Can you work these out from the drawing? Everything is in mm from the part's minimum corner. Give positions to 0.01 mm unless a question says otherwise; leave off trailing zeros. Loops run counter-clockwise (first coordinate to the right, second up) from the corner with the lowest first, then second, coordinate; pieces in that order, holes last. Notation, with made-up numbers: (-28.5, -0.75) -> (22.5, -0.75) arc R19 ccw to (22.5, 17.25) -> close; hole circle Ø7 at (6.25, -6.5). An arc over 180 degrees is marked (long way). Write item = value, one per line. Start each with the question number.
1) I need wall thicknesses on probe 1 along Y at (x, z) = (50, 52); probe 2 along Z at (x, y) = (17.5, 51.5); probe 3 along X at (y, z) = (25.5, 51) (1 decimal). Which ranges of each line are inside material? Lowest first, please. Write a range as from..to.
2) I want a section at C-C (z = 33). List the corners of the cut face in (x, y) for me.
3) If we mould it in two halves opening along Y, with no side actions, what happens to the marked faces 1, 2 and 3? For each: +Y half, -Y half, draft (parallel to the pull), parting line (faces both ways), or undercut.
4) I want a section at A-A (x = 68.5). List the corners of the cut face in (y, z) for me.
5) I'm going to push flat-ended pins straight in: pin 1 Ø8 at (y, z) = (59, 43.5) entering from -X; pin 2 Ø2 at (y, z) = (88.5, 48) entering from +X (1 decimal); pin 3 Ø10 at (y, z) = (48, 25) entering from +X; pin 4 Ø14.5 at (x, y) = (29.5, 51.5) entering from +Z. Where does each tip first touch, or does it pass through?
6) I want a section at D-D (x = 83). List the corners of the cut face in (y, z) for me.
7) I want a section at B-B (y = 82). List the corners of the cut face in (x, z) for me (1 decimal), and give its area (3 significant figures).
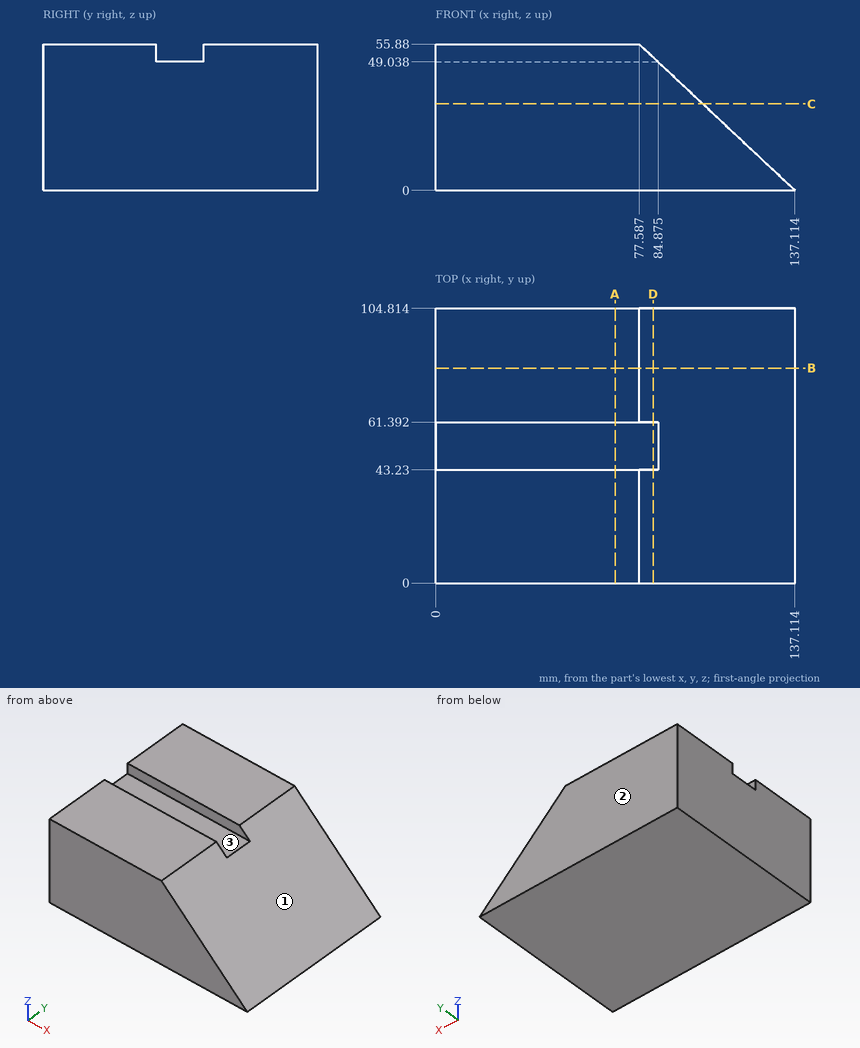
Answer list:
q1.probe_1 = 0..43.23, 61.39..104.81
q1.probe_2 = 0..49.04
q1.probe_3 = 0..82.8
q2.outline = (0, 0) -> (101.96, 0) -> (101.96, 104.81) -> (0, 104.81) -> close
q3.face_1 = draft
q3.face_2 = +Y half
q3.face_3 = undercut
q4.outline = (0, 0) -> (104.81, 0) -> (104.81, 55.88) -> (61.39, 55.88) -> (61.39, 49.04) -> (43.23, 49.04) -> (43.23, 55.88) -> (0, 55.88) -> close
q5.pin_1 = 0
q5.pin_2 = 87
q5.pin_3 = 115.81
q5.pin_4 = 49.04
q6.outline = (0, 0) -> (104.81, 0) -> (104.81, 50.8) -> (61.39, 50.8) -> (61.39, 49.04) -> (43.23, 49.04) -> (43.23, 50.8) -> (0, 50.8) -> close
q7.outline = (0, 0) -> (137.1, 0) -> (77.6, 55.9) -> (0, 55.9) -> close
q7.area = 6,000 mm^2
